Source: CAD feature listing. Evaluate the final solid. Frame: model axes, mm. A direction names the side the tool comes from. Round coordinates to 2 decimals unless told otherwise and drop trailing zeros. Order: outer loops, then holes, each group sorted by start corner. A loop starts at its lowest first (then second) coordinate and runs counter-clockwise, first axis right, second up. Notation, with made-up numbers: (-2.5, 16.25) -> (34.5, 16.25) arc R7 ccw to (34.5, 29.25) -> close; hole circle Ø10 at (-23.75, 13.25). An arc over 180 degrees is marked (long way). Answer as CSV lines item,"result". Start each with the question number.
(1) Section query C-C (y = 6.5). Output: boundary loops of the cut face in (x, z).
(2) Section query B-B (x = -0.5). Output: boundary loops of the cut face in (y, z), plus the area to 3 significant figures.
(3) Pull-direction query (X, two-part tool) for faces 1 (the cylindrical face through (16.2, 5.253, -14.777)), 2 (the cylindrical face through (15.616, 4.72, -14.923)), 3 (the flat face through (15, 0, -28.184)), 4 (the flat face through (-3.952, -6.945, -11.689)); classes: +X half, -X half, draft (parallel to the pull), parting line (faces both ways), or undercut.
(4) Section query A-A (z = -6). Output: boundary loops of the cut face in (x, y), plus the area to 3 significant figures.
(5) Line query: line 1 along X through (y, z) = (-2.75, -21); line 2 along X through (y, z) = (3.5, -26.5); line 3 along Z through (x, y) = (6, 3.5). Output: solid intervals per line, ascending. Write a range as from..to.
(6) Set-up query: faces 5 (the flat face through (-3, -8, 2)), 6 (the flat face through (3.952, 6.945, -11.689)). Return all of +Z, -Z, +X, -X, +Y, -Y with unobstructed straight access to the full face (end or side cutting, diameter ignored); none if empty.
(7) Section query D-D (x = 10.5). Output: boundary loops of the cut face in (y, z).
(8) Contact query for flat-ended pins moving along their axis: P1, Ø10, axis at x = 12.5, z = -5, coming from the -Y side; P2, Ø4, axis at x = 8.5, y = -9.5, coming from the +Z side; P3, Ø0.7, axis at x = 14.5, z = -16, coming from the +Y side; P4, Ø6, axis at y = -9, z = -9, coming from the -X side. Output: stop coordinate, or through.
```python
from build123d import *

# Parameters (mm, degrees)
F1_DEPTH = 30
F3_DEPTH = 25
F5_DEPTH = 2
F6_W     = 10.7590798289
F6_H     = 26.4430916868
F7_DEPTH = 3.5
F8_W     = 2.3892438039
F8_H     = 9.8118302412
F9_DEPTH = 26
F10_R    = 1


with BuildPart() as f1:
    # F0 (on Top) → F1 (new body)
    with BuildSketch(Plane.XY):
        Polygon((13.0044895149, 7.4755634337), (0.0282169163, 15), (-12.9762725986, 7.5244365663), (-13.0044895149, -7.4755634337), (-0.0282169163, -15), (12.9762725986, -7.5244365663), align=None)
    extrude(amount=-F1_DEPTH)

    # F2 (on face) → F3 (cut)
    with BuildSketch(Plane.XY):
        Polygon((7.9817117837, -4.6282847058), (7.999068023, 4.5982228174), (0.0173562394, 9.2265075233), (-7.9817117837, 4.6282847058), (-7.999068023, -4.5982228174), (-0.0173562394, -9.2265075233), align=None)
    extrude(amount=-F3_DEPTH, mode=Mode.SUBTRACT)

    # F4 (on face) → F5 (join)
    with BuildSketch(Plane.XY):
        Polygon((-9.9795361097, 5.78674545), (-10.0012366198, -5.7491590639), (-0.0217005101, -11.535904514), (9.9795361097, -5.78674545), (10.0012366198, 5.7491590639), (0.0217005101, 11.535904514), align=None)
        Polygon((0.0173562394, 9.2265075233), (7.999068023, 4.5982228174), (7.9817117837, -4.6282847058), (-0.0173562394, -9.2265075233), (-7.999068023, -4.5982228174), (-7.9817117837, 4.6282847058), align=None, mode=Mode.SUBTRACT)
    extrude(amount=F5_DEPTH)

    # F6 (on face) → F7 (join)
    with BuildSketch(Plane(origin=(12.9903810568, -0.0244365663, 0), x_dir=(0.0018811244, 0.9999982307, 0), z_dir=(0.9999982307, -0.0018811244, 0))):
        with Locations((0.1894203015, -14.9621136952)):
            Rectangle(F6_W, F6_H)
    extrude(amount=F7_DEPTH)

    # F8 (on face) → F9 (cut)
    with BuildSketch(Plane.XY.offset(-1.7405678518)):
        with Locations((14.7061855532, 0.1149831805)):
            Rectangle(F8_W, F8_H)
    extrude(amount=-F9_DEPTH, mode=Mode.SUBTRACT)

    # F10
    f10_edges = [f1.edges().sort_by_distance(p)[0] for p in [
        (16.480612, -5.221131, -14.962114),
        (16.500851, 5.53793, -14.962114),
        (15.900807, 5.020898, -14.740568),
        (15.900807, -4.790932, -14.740568),
    ]]
    fillet(f10_edges, radius=F10_R)


solid = f1.part
```
Answer block:
1,outline,"(-12.98, -30) -> (13, -30) -> (13, 0) -> (8.71, 0) -> (8.71, 2) -> (4.72, 2) -> (4.72, -25) -> (-4.73, -25) -> (-4.73, 2) -> (-8.74, 2) -> (-8.74, 0) -> (-12.98, 0) -> close"
2,outline,"(-14.73, -30) -> (14.7, -30) -> (14.7, 0) -> (11.24, 0) -> (11.24, 2) -> (8.93, 2) -> (8.93, -25) -> (-8.95, -25) -> (-8.95, 2) -> (-11.26, 2) -> (-11.26, 0) -> (-14.73, 0) -> close"
2,area,"445 mm2"
3,face 1,"+X half"
3,face 2,"undercut"
3,face 3,"draft"
3,face 4,"undercut"
4,outline,"(-13, -7.48) -> (-0.03, -15) -> (12.98, -7.52) -> (12.98, -5.21) -> (15.48, -5.22) arc R1 ccw to (16.48, -4.22) -> (16.5, 4.54) arc R1 ccw to (15.5, 5.54) -> (13, 5.54) -> (13, 7.48) -> (0.03, 15) -> (-12.98, 7.52) -> close; hole (-8, -4.6) -> (-0.02, -9.23) -> (7.98, -4.63) -> (8, 4.6) -> (0.02, 9.23) -> (-7.98, 4.63) -> close; hole (13.51, -4.79) -> (14.9, -4.79) arc R1 ccw to (15.9, -3.79) -> (15.9, 4.02) arc R1 ccw to (14.9, 5.02) -> (13.51, 5.02) -> close"
4,area,"378 mm2"
5,line 1,"-13..-8, 7.99..13.51, 15.9..16.49"
5,line 2,"-12.98..13.51, 15.9..16.5"
5,line 3,"-30..-25"
6,face 5,"+Z, +X, -X, +Y, -Y"
6,face 6,"+Z"
7,outline,"(-8.95, -30) -> (8.93, -30) -> (8.93, 0) -> (-8.95, 0) -> close"
8,P1,"y = -10.67"
8,P2,"z = 0"
8,P3,"y = 5.54"
8,P4,"x = -13"
